Read the model definition and answer for the solid it produces. Units are mm, in the model's axes. Face numbers are marked on the shaded views. A direction names the side the tool comes from. Round coordinates to 2 decimals unless told otherwise and drop trailing zeros. Write each loop counter-clockwise with the first axis right and the second up, starting at its lowest first coordinate (ties: lowest second). Pieces come first, ordered by that corner, then holes. Notation, with made-up numbers: (-14.75, 34) - (25.25, 34) arc R24 cw to (25.25, 53) - close; hole circle Ø4 at (28.5, -26.75). An arc over 180 degrees is marked (long way). One line per item, written item: value. Start each with the question number.
(1) The mould has two halves that part along Z. Classify the marked faces 1, 2, 3 and 4: +Z half, -Z half, draft (parallel to the pull), parting line (faces both ways), or undercut.
(2) For the marked faces 5, 6, 7, 8 and 9, determine the directions among +Z, -Z, +X, -X, +Y, -Y from which every point of the face is accessible in a straight line to the end or side of a thin tool.
(3) A cutting plane is placed at A-A, the plane z = 9.5. Determine the outline of the cut face in (x, y), plus the area to 3 significant figures.
(4) Flat-ended cylindrical pins translate along their axes: pin 1 Ø5 at (x, y) = (30, -11) entering from +Z; pin 2 Ø2 at (y, z) = (-6.5, -15.5) entering from +X; pin 3 Ø1.7 at (y, z) = (-6, 22.5) entering from +X. Find the tip coordinate at first contact, or state that the pin passes through.
(5) Find the intervals of material crossed by L1, parallel to X at y = -8.25, z = 4; L2, parallel to Y at x = 19.5, z = -1; L3, parallel to X at y = -3.25, z = -21, in increasing order.
(6) A cutting plane is placed at B-B, the plane x = -6.5. Determine the outline of the cut face in (y, z), plus the area to 3 significant figures.
(7) A cutting plane is placed at C-C, the plane y = -23.25. Determine the outline of the cut face in (x, z).
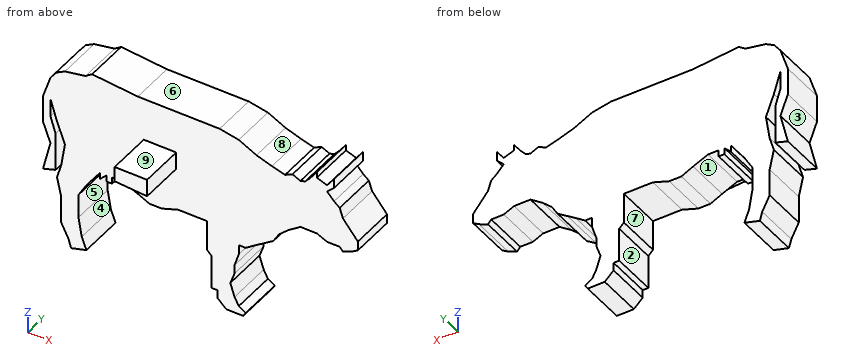
from build123d import *

# Parameters (mm, degrees)
F1_DEPTH = 12.7
F3_DEPTH = 12.7


with BuildPart() as f1:
    # F0 (on Front) → F1 (new body)
    with BuildSketch(Plane.XZ):
        Polygon((-28.615356, 25.77387), (-30.462335, 24.485242), (-36.267126, 23.429823), (-38.641814, 22.110556), (-40.356866, 19.867797), (-42.461474, 13.535295), (-42.461474, 5.883527), (-40.356866, 0.342589), (-42.461474, -8.147422), (-38.919031, -7.045326), (-38.919031, -0.844754), (-38.919031, 3.768534), (-40.356866, 8.39014), (-40.356866, 13.535295), (-38.509885, 7.598579), (-36.267126, 1.66186), (-37.322543, -5.06642), (-38.509885, -9.024232), (-37.322543, -14.433242), (-37.322543, -22.085012), (-35.219288, -26.17475), (-34.552074, -28.573201), (-30.19848, -27.362095), (-31.517752, -23.931991), (-32.441241, -18.522981), (-32.441241, -11.794701), (-30.19848, -7.968816), (-26.372596, -2.691734), (-26.372596, -4.538711), (-24.525617, -2.691734), (-24.525617, -4.538711), (-22.942492, -4.538711), (-22.942492, -2.691734), (-19.90817, -2.691734), (-15.686504, -4.538711), (-12.388325, -6.121836), (-8.958223, -6.121836), (-4.340774, -4.538711), (0.012816, -4.538711), (3.838704, -4.538711), (3.838704, -7.968816), (3.838704, -13.113971), (5.157971, -14.433242), (5.157971, -18.522981), (5.157971, -23.931991), (6.741096, -23.931991), (6.741096, -26.17475), (9.24771, -28.573201), (14.061987, -28.573201), (14.788651, -27.362095), (12.809743, -26.17475), (11.6224, -23.931991), (10.435057, -20.238034), (11.6224, -16.939856), (11.6224, -14.433242), (12.809743, -10.739285), (12.809743, -7.968816), (14.788651, -7.968816), (17.427192, -6.121836), (19.801878, -4.538711), (22.572347, -2.691734), (24.155469, -0.053193), (26.79401, 2.321497), (30.224116, 4.696183), (32.862657, 4.696183), (34.841561, 4.696183), (37.743957, 3.376913), (41.30599, 3.376913), (42.229482, 2.321497), (44.736096, 3.376913), (46.438526, 4.432328), (46.438526, 7.07087), (42.229482, 12.216028), (41.30599, 14.986497), (39.722868, 16.296333), (37.743957, 18.416595), (39.722868, 20.263579), (39.722868, 22.90212), (37.743957, 20.263579), (34.841561, 21.318991), (34.841561, 22.90212), (32.862657, 20.263579), (31.543382, 18.812377), (30.224116, 18.416595), (27.981357, 19.472015), (25.870525, 18.416595), (22.176565, 19.472015), (17.822974, 20.923209), (12.809743, 23.429823), (7.400733, 24.485242), (0.144743, 24.485242), (-8.298586, 24.485242), (-15.686504, 24.485242), align=None)
    extrude(amount=F1_DEPTH)

    # F2 (on face) → F3 (join)
    with BuildSketch(Plane.XZ.offset(12.7)):
        Polygon((-14.009252, 12.325057), (-14.009252, 8.07736), (-4.843168, 7.406671), (-4.843168, 12.325057), align=None)
    extrude(amount=F3_DEPTH)


solid = f1.part
Here are the results:
1. face 1: -Z half
1. face 2: draft
1. face 3: undercut
1. face 4: undercut
2. face 5: +Y, -Y
2. face 6: +Z, +X, +Y, -Y
2. face 7: -Z, +Y, -Y
2. face 8: +Z, +Y, -Y
2. face 9: +Z, +X, -X, -Y
3. outline: (-42.46, -12.7) - (-40.36, -12.7) - (-40.36, 0) - (-42.46, 0) - close; (-39.1, -12.7) - (-14.01, -12.7) - (-14.01, -25.4) - (-4.84, -25.4) - (-4.84, -12.7) - (44.45, -12.7) - (44.45, 0) - (-39.1, 0) - close
3. area: 1,200 mm²
4. pin 1: z = 19.86
4. pin 2: x = 11.62
4. pin 3: x = 39.72
5. L1: -41.75 to -38.99, -37.15 to 29.22, 36.37 to 45.74
5. L2: -12.7 to 0
5. L3: -37.32 to -32.02, 5.16 to 10.68
6. outline: (-25.4, 7.53) - (-12.7, 7.53) - (-12.7, -5.28) - (0, -5.28) - (0, 24.49) - (-12.7, 24.49) - (-12.7, 12.33) - (-25.4, 12.33) - close
6. area: 439 mm²
7. outline: (-14.01, 8.08) - (-4.84, 7.41) - (-4.84, 12.33) - (-14.01, 12.33) - close
